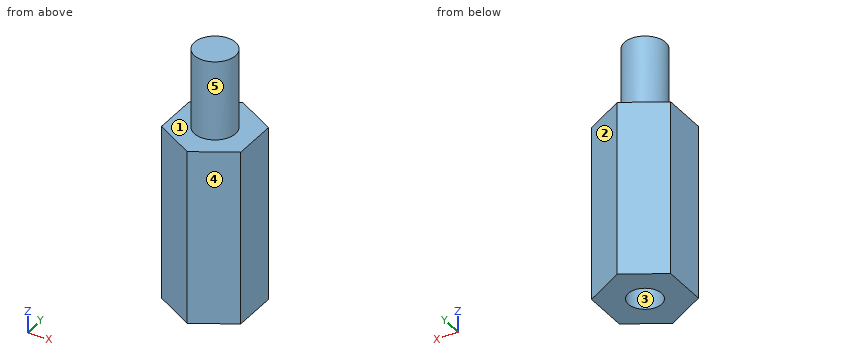
Autodesk Inventor part; units mm, degrees
ref_plane "YZ Plane" through (0, 0, 0) normal (1, 0, 0) x (0, 1, 0)
ref_plane "XZ Plane" through (0, 0, 0) normal (0, 1, 0) x (-1, 0, 0)
ref_plane "XY Plane" through (0, 0, 0) normal (0, 0, 1) x (1, 0, 0)
sketch "スケッチ1" plane through (0, 0, 0) normal (0, 0, 1) x (1, 0, 0)
  line L0 (0, 2.8868) -> (2.5, 1.4434)
  line L1 (2.5, 1.4434) -> (2.5, -1.4434)
  line L2 (2.5, -1.4434) -> (0, -2.8868)
  line L3 (0, -2.8868) -> (-2.5, -1.4434)
  line L4 (-2.5, -1.4434) -> (-2.5, 1.4434)
  line L5 (-2.5, 1.4434) -> (0, 2.8868)
  point P0 (0, 0)
  point P1 (0, 0)
  dimension "d0" = 5
extrude "押し出し1" add sketch "スケッチ1" along normal blind 11
sketch "スケッチ2" plane through (0, 0, 11) normal (0, 0, 1) x (1, 0, 0)
  circle A0 centre (0, 0) radius 1.3
  dimension "d3" = 2.6
extrude "押し出し2" add sketch "スケッチ2" along normal blind 5
thread "ねじ1"
sketch "スケッチ3" plane through (0, 0, 0) normal (0, 0, -1) x (-1, 0, 0)
  point P0 (0, 0)
hole "穴1" at (0, 0, 0) direction (0, 0, 1) diameter 2.113 depth 7.8 tip angle 118
properties part number "ジュラコンスペーサー（六角）_BS-2611E" material "アセタール樹脂、白"
Geometry check sheet. Reference: the model listing, model coordinates, mm. Face numbers are marked on the shaded views. A direction names the side the tool comes from. Round coordinates to 2 decimals unless told otherwise and drop trailing zeros. Write each loop counter-clockwise with the first axis right and the second up, starting at its lowest first coordinate (ties: lowest second). Pieces come first, ordered by that corner, then holes. Notation, with made-up numbers: (23.5, 1.25) - (77.5, 1.25) arc R19 cw to (77.5, 25.25) - close; hole circle Ø2 at (-12.5, -11). An arc over 180 degrees is marked (long way). One line per item, written item: value.
1. Cross-section at B-B on z = 9.75. Record the boundary of the cut face in (x, y).
The answers:
outline: (-2.5, -1.44) - (0, -2.89) - (2.5, -1.44) - (2.5, 1.44) - (0, 2.89) - (-2.5, 1.44) - close
2. Mould release check, pull along Y, two halves, no side actions. Record for the marked faces 3, 4 and 5: released by +Y, released by -Y, zero draft, split by the parting line, or undercut.
The answers:
face 3: undercut
face 4: released by -Y
face 5: split by the parting line
3. Depth check by flat-ended pin: pin 1 Ø1.5 at (x, z) = (-1, 5.5) entering from -Y; pin 2 Ø1 at (y, z) = (-0.5, 12.5) entering from -X; pin 3 Ø2 at (x, z) = (2, 7) entering from -Y. Enter the tip coordinate at first touch or a pass-through.
The answers:
pin 1: stops at y = -2.74
pin 2: stops at x = -1.3
pin 3: stops at y = -2.31
4. Cross-section at A-A on z = 6.75. Record the boundary of the cut face in (x, y), and give its area (3 significant figures).
The answers:
outline: (-2.5, -1.44) - (0, -2.89) - (2.5, -1.44) - (2.5, 1.44) - (0, 2.89) - (-2.5, 1.44) - close; hole circle Ø2.11 at (0, 0)
area: 18.1 mm^2
5. Scan lines: L1, parallel to X at y = 0, z = 2.25; L2, parallel to Z at x = 1.8, y = -0.9; L3, parallel to Y at x = 0.25, z = 6.25. Record each from-to range of solid material in increasing order.
The answers:
L1: x = -2.5 to -1.06, 1.06 to 2.5
L2: z = 0 to 11
L3: y = -2.74 to -1.03, 1.03 to 2.74
6. Cross-section at C-C on y = -2.45. Record the boundary of the cut face in (x, z), and give its area (3 significant figures).
The answers:
outline: (-0.76, 0) - (0.76, 0) - (0.76, 11) - (-0.76, 11) - close
area: 16.6 mm^2
7. Set-up check for the marked faces 1 and 2: record each of +Z, -Z, +X, -X, +Y, -Y from which the full face is reachable in a straight line by a thin tool's end or side.
The answers:
face 1: +Z
face 2: +Z, -Z, +X, +Y
8. Cross-section at D-D on x = -1.75. Record the boundary of the cut face in (y, z), and give its area (3 significant figures).
The answers:
outline: (-1.88, 0) - (1.88, 0) - (1.88, 11) - (-1.88, 11) - close
area: 41.3 mm^2
